```python
from build123d import *

# Parameters (mm, degrees)
PAD016_DEPTH         = 9.7
SKETCH041_R          = 1.65
POCKET014_DEPTH      = 0.001
POCKET014_DEPTH_BACK = 8.501
SKETCH042_W          = 5.8
SKETCH042_H          = 2.7
POCKET015_DEPTH      = 8.3


with BuildPart() as part:
    # Sketch040 → Pad016 (new body)
    with BuildSketch(Plane.XY):
        with BuildLine():
            ThreePointArc((5.05198, -8.5), (0, -4.35), (-5.05198, -8.5))
            Line((-14, -8.5), (-5.05198, -8.5))
            Line((-14, -0.5), (-14, -8.5))
            Line((-14, -0.5), (14, -0.5))
            Line((14, -0.5), (14, -8.5))
            Line((14, -8.5), (5.05198, -8.5))
        make_face()
    extrude(amount=PAD016_DEPTH)

    # Sketch041 → Pocket014 (cut, two sides)
    with BuildSketch(Plane.XZ) as pocket014_sk:
        with Locations((-8.02599, 5)):
            Circle(SKETCH041_R)
        with Locations((8.02599, 5)):
            Circle(SKETCH041_R)
    extrude(amount=-POCKET014_DEPTH, mode=Mode.SUBTRACT)
    extrude(pocket014_sk.sketch, amount=POCKET014_DEPTH_BACK, mode=Mode.SUBTRACT)

    # Sketch042 (on Face4 of Pocket014) → Pocket015 (cut)
    with BuildSketch(Plane.XY.offset(9.7)):
        with Locations((-8.02599, -3.85)):
            Rectangle(SKETCH042_W, SKETCH042_H)
    pocket015 = extrude(amount=-POCKET015_DEPTH, mode=Mode.SUBTRACT)

    # Mirrored001: Pocket015 across Sketch042 V_Axis
    add(pocket015.mirror(Plane(origin=(0, 0, 9.7), x_dir=(0, 0, 1), z_dir=(1, 0, 0))), mode=Mode.SUBTRACT)


solid = part.part
```
CAD build for the part. Positions are in the model's coordinates, mm. A direction names the side the tool comes from. Coordinates: 2 decimals unless noted, no trailing zeros. Order: outer loops, then holes, each group sorted by start corner. A loop starts at its lowest first (then second) coordinate and runs counter-clockwise, first axis right, second up. Notation, with made-up numbers: (-7, -34) - (2, -34) arc R17 ccw to (2, -3) - close; hole circle Ø1 at (37, 27). An arc over 180 degrees is marked (long way). Answer in a Markdown table with one row per item.
1. 3-axis set-ups, long thin cutter, end or side, ignore diameter. For faces 1 (the face through (-7.26, -6.83, 3.54)), 2 (the face through (5.126, -4, 6)): which of +Z, -Z, +X, -X, +Y, -Y reach the whole face in a straight line?
Answer:
| item | result |
|---|---|
| face 1 | +Y, -Y |
| face 2 | +Z |
2. Flat gauge pins, fed straight in: P1, Ø2, axis at x = 8, y = -4, coming from the +Z side; P2, Ø1.7, axis at x = -8.5, z = 5, coming from the +Y side; P3, Ø3, axis at x = -3, z = 8, coming from the -Y side. Where does each tip first touch, or does it go through?
Answer:
| item | result |
|---|---|
| P1 | z = 1.4 |
| P2 | through |
| P3 | y = -7 |
3. Slice it at A-A, the plane y = -8. List the corners of the cut face in (x, z).
Answer:
| item | result |
|---|---|
| outline | (-14, 0) - (-4.93, 0) - (-4.93, 9.7) - (-14, 9.7) - close; (4.93, 0) - (14, 0) - (14, 9.7) - (4.93, 9.7) - close; hole circle Ø3.3 at (-8.03, 5); hole circle Ø3.3 at (8.03, 5) |
4. Slice it at D-D, the plane x = -6. List the corners of the cut face in (y, z).
Answer:
| item | result |
|---|---|
| outline | (-8.5, 0) - (-0.5, 0) - (-0.5, 9.7) - (-2.5, 9.7) - (-2.5, 1.4) - (-5.2, 1.4) - (-5.2, 9.7) - (-8.5, 9.7) - close |
5. Pull direction X, two halves, no side cores. Call faces 3 (the face through (-10.926, -4, 6)), 4 (the face through (14, -4, 5)), 5 (the face through (-14, -4, 5)), 6 (the face through (0, -4, 0)): +X half, -X half, draft (parallel to the pull), parting line (faces both ways), or undercut.
Answer:
| item | result |
|---|---|
| face 3 | undercut |
| face 4 | +X half |
| face 5 | -X half |
| face 6 | draft |
6. Slice it at C-C, the plane z = 5. Give the number of separate pieces and of enclosed holes in the cut face, then the cut area to 3 significant figures.
Answer:
| item | result |
|---|---|
| separate pieces | 3 |
| enclosed holes | 0 |
| area | 126 mm² |
7. Slice it at B-B, the plane z = 3. List the corners of the cut face in (x, y), then the cut area to 3 significant figures.
Answer:
| item | result |
|---|---|
| outline | (-14, -8.5) - (-5.05, -8.5) arc R5.15 cw to (5.05, -8.5) - (14, -8.5) - (14, -0.5) - (-14, -0.5) - close; hole (-10.93, -5.2) - (-5.13, -5.2) - (-5.13, -2.5) - (-10.93, -2.5) - close; hole (5.13, -5.2) - (10.93, -5.2) - (10.93, -2.5) - (5.13, -2.5) - close |
| area | 161 mm² |
8. Drill centre lines: L1, parallel to X at y = -3.75, z = 6.25; L2, parallel to X at y = -1.45, z = 5; L3, parallel to Y at x = -5.5, z = 5. Where is each one in solid material? Low to high. Write a range as from..to.
Answer:
| item | result |
|---|---|
| L1 | -14..-10.93, -5.13..5.13, 10.93..14 |
| L2 | -14..-9.68, -6.38..6.38, 9.68..14 |
| L3 | -8.5..-5.2, -2.5..-0.5 |
